from build123d import *
from build123d.topology import SkipClean

# Parameters (mm, degrees)
SKETCH1_R           = 25
SKETCH1_R_2         = 2.5
BOSS_EXTRUDE1_DEPTH = 5
SKETCH2_R           = 2.5
BOSS_EXTRUDE2_DEPTH = 5
BOSS_EXTRUDE3_START = 5
SKETCH3_R           = 2.5
BOSS_EXTRUDE3_DEPTH = 5
BOSS_EXTRUDE4_START = 35
SKETCH4_R           = 5
SKETCH4_R_2         = 2.5
BOSS_EXTRUDE4_DEPTH = 35
BOSS_EXTRUDE5_START = -50
SKETCH5_R           = 2.5
BOSS_EXTRUDE5_DEPTH = 55
SKETCH6_W           = 3.535533906
SKETCH6_H           = 3.535533906
BOSS_EXTRUDE6_DEPTH = 5


with BuildPart() as part:
    # Sketch1 → Boss-Extrude1 (new body)
    with BuildSketch(Plane(origin=(0, 0, 0), x_dir=(1, 0, 0), z_dir=(0, 1, 0))):
        with Locations(Location((0, 0, 0), (0, 0, 270))):
            Circle(SKETCH1_R)
        with Locations(Location((0, 0, 0), (0, 0, 270))):
            Circle(SKETCH1_R_2, mode=Mode.SUBTRACT)
    extrude(amount=BOSS_EXTRUDE1_DEPTH)

    # Sketch2 → Boss-Extrude2 (add)
    with BuildSketch(Plane.XZ):
        with Locations(Location((0, 22.5, 0), (0, 0, 90))):
            Circle(SKETCH2_R)
    extrude(amount=BOSS_EXTRUDE2_DEPTH)

    # Sketch3 → Boss-Extrude3 (add)
    with SkipClean():  # the faces are left unmerged after this step: merging them gives an invalid solid
        with BuildSketch(Plane.XZ.offset(BOSS_EXTRUDE3_START)):
            with BuildLine():
                ThreePointArc((-12.29868157, 10.234375), (0, -16), (12.29868157, 10.234375))
                ThreePointArc((12.29868157, 10.234375), (0, 7), (-12.29868157, 10.234375))
            make_face()
            with Locations(Location((0, 0, 0), (0, 0, 270))):
                Circle(SKETCH3_R, mode=Mode.SUBTRACT)
        extrude(amount=-BOSS_EXTRUDE3_DEPTH)

    # Sketch4 → Boss-Extrude4 (add)
    with SkipClean():  # the faces are left unmerged after this step: merging them gives an invalid solid
        with BuildSketch(Plane.XZ.offset(5).offset(BOSS_EXTRUDE4_START)):
            with Locations(Location((0, 0, 0), (0, 0, 270))):
                Circle(SKETCH4_R)
            with Locations(Location((0, 0, 0), (0, 0, 270))):
                Circle(SKETCH4_R_2, mode=Mode.SUBTRACT)
        extrude(amount=-BOSS_EXTRUDE4_DEPTH)

    # Sketch5 → Boss-Extrude5 (add)
    with BuildSketch(Plane(origin=(0, 5, 0), x_dir=(1, 0, 0), z_dir=(0, 1, 0)).offset(BOSS_EXTRUDE5_START)):
        with Locations(Location((0, 0, 0), (0, 0, 90))):
            Circle(SKETCH5_R)
    extrude(amount=BOSS_EXTRUDE5_DEPTH)

    # Sketch6 → Boss-Extrude6 (add)
    with BuildSketch(Plane(origin=(0, 10, 0), x_dir=(1, 0, 0), z_dir=(0, 1, 0))):
        Rectangle(SKETCH6_W, SKETCH6_H)
    extrude(amount=BOSS_EXTRUDE6_DEPTH)


solid = part.part
Work out the finished part from the listing and answer in its coordinate system (mm). A direction names the side the tool comes from. Coordinates: 2 decimals unless noted, no trailing zeros. Order: outer loops, then holes, each group sorted by start corner. A loop starts at its lowest first (then second) coordinate and runs counter-clockwise, first axis right, second up. Notation, with made-up numbers: (12, -20) - (57, -20) arc R10 cw to (57, -14) - close; hole circle Ø6 at (-21, -37.5). An arc over 180 degrees is marked (long way). Put each result on its own line as item: value. Start each with the question number.
1) Find section C-C (y = -22). Give the vertices of the cut face in (x, z).
2) For a pull along Z with two mould halves and no side action, classify faces 5 (the cylindrical face through (2.44, 7.47, 0.54)), 6 (the flat face through (1.768, 12, 0)), 7 (the cylindrical face through (0, -2, 20)) as released by +Z, released by -Z, zero draft, split by the parting line, or undercut.
3) For faces 1 (the flat face through (0, 12, 1.768)), 2 (the flat face through (0, 12, -1.768)), 3 (the cylindrical face through (2.44, -42.54, 0.54)), 4 (the flat face through (0, -5, 22)), determine the directions among +Z, -Z, +X, -X, +Y, -Y from which every point of the face is accessible in a straight line to the end or side of a thin tool.
4) Flat-ended cylindrical pins translate along their axes: pin 1 (6 mm diameter, centred on x = 9, z = 3, fed in from -Y); pin 2 (1 mm diameter, centred on x = 9, z = -11.5, fed in from +Y); pin 3 (25 mm diameter, centred on x = 11.5, z = -9.5, fed in from -Y); pin 4 (1.5 mm diameter, centred on x = -6.5, y = 1.5, fed in from -Z). Find the tip coordinate at first contact, or state that the pin passes through.
5) Find section D-D (z = 22.5). Give the vertices of the cut face in (x, y), plus the area to 3 significant figures.
6) Find section A-A (z = 0). Give the vertices of the cut face in (x, y).
7) Find the intervals of material crossed by line 1 (Y direction, x = 11, z = 14); line 2 (Y direction, x = -9.5, z = 8.5); line 3 (Z direction, x = -12, y = -3), in increasing order. Write a range as from..to.
8) Find section B-B (x = 9). Give the vertices of the cut face in (y, z).
Results list:
1. outline: circle Ø10 at (0, 0)
2. face 5: split by the parting line
2. face 6: zero draft
2. face 7: undercut
3. face 1: +Z, +X, -X, +Y
3. face 2: -Z, +X, -X, +Y
3. face 3: -Y
3. face 4: +Z, +X, -X, -Y
4. pin 1: stops at y = -5
4. pin 2: stops at y = 5
4. pin 3: stops at y = -45
4. pin 4: stops at z = -24.33
5. outline: (-10.9, 0) - (-2.5, 0) - (-2.5, -5) - (2.5, -5) - (2.5, 0) - (10.9, 0) - (10.9, 5) - (-10.9, 5) - close
5. area: 134 mm^2
6. outline: (-25, 0) - (-16, 0) - (-16, -5) - (-5, -5) - (-5, -40) - (-2.5, -40) - (-2.5, -45) - (2.5, -45) - (2.5, -40) - (5, -40) - (5, -5) - (16, -5) - (16, 0) - (25, 0) - (25, 5) - (2.5, 5) - (2.5, 10) - (1.77, 10) - (1.77, 15) - (-1.77, 15) - (-1.77, 10) - (-2.5, 10) - (-2.5, 5) - (-25, 5) - close
7. line 1: y = 0..5
7. line 2: y = -5..5
7. line 3: z = -10.58..10.07
8. outline: (-5, -13.23) - (0, -13.23) - (0, -23.32) - (5, -23.32) - (5, 23.32) - (0, 23.32) - (0, 8.68) - (-5, 8.68) - close
